```python
from build123d import *

# Parameters (mm, degrees)
SKETCH1_R                      = 2.4257
EXTRUDE1_DEPTH                 = 0.381
SKETCH2_W                      = 2.286
SKETCH2_H                      = 1.0668
EB_02_TAB_1_DEPTH              = 0.381
LP_01_TAB_1_X_29_X_0_600_COUNT = 29
LP_01_TAB_1_X_29_X_0_600_PITCH = 15.24
SKETCH5_W                      = 6.469789446
SKETCH5_H                      = 8.753244544
EXTRUDE5_DEPTH                 = 0.254


with BuildPart() as part:
    # Sketch1 → Extrude1 (new, symmetric)
    with BuildSketch(Plane.XY):
        Polygon((128.4732, 0), (566.7248, 0), (562.825597202, -22.113477941), (128.4732, -5.047725776), align=None)
        with Locations(Location((552.014887855, -10.287672178, 0), (0, 0, 180))):
            Circle(SKETCH1_R, mode=Mode.SUBTRACT)
    extrude(amount=EXTRUDE1_DEPTH, both=True)

    # Sketch2 → EB-02 Tab 1 (add, symmetric)
    with BuildSketch(Plane.XY):
        with Locations((133.223, 0.2794)):
            Rectangle(SKETCH2_W, SKETCH2_H)
    eb_02_tab_1 = extrude(amount=EB_02_TAB_1_DEPTH, both=True)

    # LP-01 Tab 1 x 29 x 0.600: EB-02 Tab 1 ×29
    with Locations(*[(i * LP_01_TAB_1_X_29_X_0_600_PITCH, 0, 0) for i in range(1, LP_01_TAB_1_X_29_X_0_600_COUNT)]):
        add(eb_02_tab_1)

    # Sketch5 → Extrude5 (cut)
    with BuildSketch(Plane.XY.offset(0.381)):
        with Locations((128.286305277, -2.289052867)):
            Rectangle(SKETCH5_W, SKETCH5_H)
    extrude(amount=-EXTRUDE5_DEPTH, mode=Mode.SUBTRACT)


solid = part.part
```
Model file for the job. Use its own axes, mm. Give positions to 0.01 mm unless a question says otherwise; leave off trailing zeros. Loops run counter-clockwise (first coordinate to the right, second up) from the corner with the lowest first, then second, coordinate; pieces in that order, holes last. Notation, with made-up numbers: (74, 56) - (81, 56) arc R18 cw to (81, 86) - close; hole circle Ø6 at (-8, 77). An arc over 180 degrees is marked (long way). One line per item, written item: value. Start each with the question number.
1. Slice it at A-A (x = 458). List the corners of the cut face in (y, z), plus the area to 3 significant figures.
2. Slice it at B-B (y = -16.5). List the corners of the cut face in (x, z).
3. Probe L1, parallel to Y at x = 436.5, z = 0.15; L2, parallel to Y at x = 156.5, z = -0.25; L3, parallel to X at y = -4.5, z = 0.3. List the from-to ranges inside material, lowest first. Write a range as from..to.
Solution:
1. outline: (-17.99, -0.38) - (0, -0.38) - (0, 0.38) - (-17.99, 0.38) - close
1. area: 13.7 mm^2
2. outline: (419.95, -0.38) - (563.82, -0.38) - (563.82, 0.38) - (419.95, 0.38) - close
3. L1: y = -17.15..0
3. L2: y = -6.15..0
3. L3: x = 131.52..565.93
